```python
from build123d import *

# Parameters (mm, degrees)
SALIENTE_EXTRUIR1_DEPTH = 8
CROQUIS2_W              = 6.524931815
CROQUIS2_H              = 4.893891774
SALIENTE_EXTRUIR2_DEPTH = 25


with BuildPart() as part:
    # Croquis1 → Saliente-Extruir1 (new body)
    with BuildSketch(Plane(origin=(0, 0, 0), x_dir=(1, 0, 0), z_dir=(0, 1, 0))):
        with BuildLine():
            Line((-23.998421012, 0), (-23.998421012, -40.04621649))
            ThreePointArc((-23.998421012, -40.04621649), (0, -64.044637502), (23.998421012, -40.04621649))
            Line((23.998421012, -40.04621649), (23.998421012, 0))
            Line((23.998421012, 0), (0, 0))
            Line((0, 0), (-23.998421012, 0))
        make_face()
    extrude(amount=SALIENTE_EXTRUIR1_DEPTH)

    # Croquis2 → Saliente-Extruir2 (add)
    with BuildSketch(Plane(origin=(0, 0, 0), x_dir=(-1, 0, 0), z_dir=(0, 0, -1))):
        with Locations((-0.697117267, 4.775150066)):
            Rectangle(CROQUIS2_W, CROQUIS2_H)
    extrude(amount=SALIENTE_EXTRUIR2_DEPTH)


solid = part.part
```
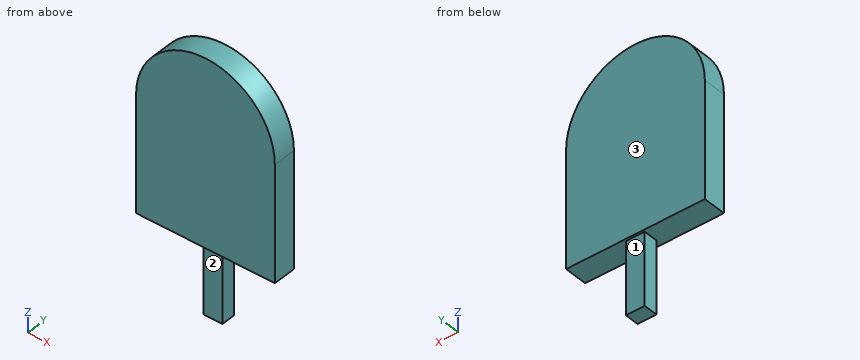
The listing builds one solid part. Answer for the finished solid, in the listing's coordinates (mm). Face numbers are marked on the shaded views. A direction names the side the tool comes from. Give positions to 0.01 mm unless a question says otherwise; leave off trailing zeros. Order: outer loops, then holes, each group sorted by start corner. A loop starts at its lowest first (then second) coordinate and runs counter-clockwise, first axis right, second up. Notation, with made-up numbers: (85, -15) - (115, -15) arc R23 ccw to (115, 13) - close; hole circle Ø1 at (-29, 75.5). An arc over 180 degrees is marked (long way). Use one line per item in the form item = value. Start each with the question number.
(1) A cutting plane is placed at B-B, the plane x = 0. Write down the section's boundary in (y, z).
(2) Consider line 1 (Z direction, x = 0, y = 6.5); line 2 (X direction, y = 4, z = -20.5); line 3 (X direction, y = 3.5, z = 49). Determine where each line is inside the solid, lowest interval first. Write a range as from..to.
(3) A cutting plane is placed at C-C, the plane z = -9. Write down the section's boundary in (x, y).
(4) A cutting plane is placed at D-D, the plane x = -20.5. Write down the section's boundary in (y, z), then the cut area to 3 significant figures.
(5) A cutting plane is placed at A-A, the plane y = 5. Write down the section's boundary in (x, z), then the cut area to 3 significant figures.
(6) For the marked faces 1, 2 and 3, determine the directions among +Z, -Z, +X, -X, +Y, -Y from which every point of the face is accessible in a straight line to the end or side of a thin tool.
(7) Flat-ended cylindrical pins translate along their axes: pin 1 Ø4 at (x, y) = (-8.5, 4) entering from -Z; pin 2 Ø3 at (y, z) = (2.5, 54.5) entering from -X; pin 3 Ø4 at (y, z) = (4.5, -15) entering from +X. Find the tip coordinate at first contact, or state that the pin passes through.
Ans:
q1.outline = (0, 0) - (2.33, 0) - (2.33, -25) - (7.22, -25) - (7.22, 0) - (8, 0) - (8, 64.04) - (0, 64.04) - close
q2.line_1 = -25..64.04
q2.line_2 = -2.57..3.96
q2.line_3 = -22.27..22.27
q3.outline = (-2.57, 2.33) - (3.96, 2.33) - (3.96, 7.22) - (-2.57, 7.22) - close
q4.outline = (0, 0) - (8, 0) - (8, 52.52) - (0, 52.52) - close
q4.area = 420 mm^2
q5.outline = (-24, 0) - (-2.57, 0) - (-2.57, -25) - (3.96, -25) - (3.96, 0) - (24, 0) - (24, 40.05) arc R24 ccw to (-24, 40.05) - close
q5.area = 2,990 mm^2
q6.face_1 = -Z, +X, -X, +Y
q6.face_2 = -Z, +X, -X, -Y
q6.face_3 = +Z, -Z, +X, -X, +Y
q7.pin_1 = 0
q7.pin_2 = -20.2
q7.pin_3 = 3.96
